```python
from build123d import *

# Parameters (mm, degrees)
BOSS_EXTRUDE1_DEPTH = 14
SKETCH2_R           = 2.75
CUT_EXTRUDE1_DEPTH  = 33.9


with BuildPart() as part:
    # Sketch1 → Boss-Extrude1 (new body)
    with BuildSketch(Plane.XY):
        with BuildLine():
            Line((-20.85, 6), (-20.85, 0))
            Line((-20.85, 0), (20.85, 0))
            Line((20.85, 0), (20.85, 6))
            Line((20.85, 6), (9, 6))
            Line((9, 6), (9, 32.9))
            Line((9, 32.9), (0.2, 32.9))
            Line((0.2, 32.9), (0.2, 24.445177921))
            ThreePointArc((0.2, 24.445177921), (3.004371815, 23.162909359), (4.15, 20.3))
            ThreePointArc((4.15, 20.3), (-2.862909359, 17.295628185), (-0.2, 24.445177921))
            Line((-0.2, 24.445177921), (-0.2, 32.9))
            Line((-0.2, 32.9), (-9, 32.9))
            Line((-9, 32.9), (-9, 6))
            Line((-9, 6), (-20.85, 6))
        make_face()
    extrude(amount=BOSS_EXTRUDE1_DEPTH)

    # Sketch2 → Cut-Extrude1 (cut, through all)
    with BuildSketch(Plane.XZ):
        with Locations((-15.85, 7)):
            Circle(SKETCH2_R)
        with Locations((15.85, 7)):
            Circle(SKETCH2_R)
    extrude(amount=-CUT_EXTRUDE1_DEPTH, mode=Mode.SUBTRACT)


solid = part.part
```
Read the model definition and answer for the solid it produces. Units are mm, in the model's axes. A direction names the side the tool comes from. Give positions to 0.01 mm unless a question says otherwise; leave off trailing zeros. Write each loop counter-clockwise with the first axis right and the second up, starting at its lowest first coordinate (ties: lowest second). Pieces come first, ordered by that corner, then holes. Notation, with made-up numbers: (32, -26) -> (90, -26) arc R18 ccw to (90, -9) -> close; hole circle Ø3 at (7, 0). An arc over 180 degrees is marked (long way). Answer in a Markdown table with one row per item.
1) A tool of negligible diameter and unlimited length cuts with its end or side. For faces 1 (the flat face through (0, 0, 7)), 2 (the flat face through (9, 19, 7)), 3 (the flat face through (-0.2, 29, 7)), 4 (the flat face through (-13.5, 6, 5.3)), from which of +Z, -Z, +X, -X, +Y, -Y can it reach the whole face along a straight path? Write none if from no direction.
Results list:
| item | result |
|---|---|
| face 1 | +Z, -Z, +X, -X, -Y |
| face 2 | +Z, -Z, +X, +Y |
| face 3 | +Z, -Z, +Y |
| face 4 | +Z, -Z, -X, +Y |
2) Each of these flat-tipped pins is pushed along its axis until it touches: pin 1 Ø4 at (y, z) = (28.5, 4) entering from -X; pin 2 Ø7 at (y, z) = (30, 7) entering from +X; pin 3 Ø3.5 at (x, z) = (-15.5, 9) entering from +Y. Where does it stop, or does it pass through?
Results list:
| item | result |
|---|---|
| pin 1 | x = -9 |
| pin 2 | x = 9 |
| pin 3 | y = 6 |
3) Section B-B on x = -15.85 is taken. Give the vertices of the cut face in (y, z).
Results list:
| item | result |
|---|---|
| outline | (0, 0) -> (6, 0) -> (6, 4.25) -> (0, 4.25) -> close; (0, 9.75) -> (6, 9.75) -> (6, 14) -> (0, 14) -> close |
4) Section C-C on z = 3 is taken. Give the vertices of the cut face in (x, y).
Results list:
| item | result |
|---|---|
| outline | (-20.85, 0) -> (20.85, 0) -> (20.85, 6) -> (9, 6) -> (9, 32.9) -> (0.2, 32.9) -> (0.2, 24.45) arc R4.15 cw (long way) to (-0.2, 24.45) -> (-0.2, 32.9) -> (-9, 32.9) -> (-9, 6) -> (-20.85, 6) -> close |
5) Straight lines are drawn through the part: line 1 (X direction, y = 25.5, z = 0.75); line 2 (Z direction, x = 15.85, y = 3.25); line 3 (Y direction, x = 0, z = 8.75). For each, find the intervals that lie inside material, in ascending order. Write a range as [from, to].
Results list:
| item | result |
|---|---|
| line 1 | [-9, -0.2], [0.2, 9] |
| line 2 | [0, 4.25], [9.75, 14] |
| line 3 | [0, 16.15] |
6) Section D-D on y = 13.5 is taken. Give the vertices of the cut face in (x, z).
Results list:
| item | result |
|---|---|
| outline | (-9, 0) -> (9, 0) -> (9, 14) -> (-9, 14) -> close |
7) Section A-A on y = 29.5 is taken. Give the vertices of the cut face in (x, z).
Results list:
| item | result |
|---|---|
| outline | (-9, 0) -> (-0.2, 0) -> (-0.2, 14) -> (-9, 14) -> close; (0.2, 0) -> (9, 0) -> (9, 14) -> (0.2, 14) -> close |
8) Determine the mould class of faces 5 (the flat face through (-5, 32.9, 7)), 6 (the flat face through (20.85, 3, 7)), 7 (the cylindrical face through (18.39, 2.96, 5.95)), 8 (the flat face through (-9, 20, 7)) for opening direction X: released by +X, released by -X, zero draft, split by the parting line, or undercut.
Results list:
| item | result |
|---|---|
| face 5 | zero draft |
| face 6 | released by +X |
| face 7 | undercut |
| face 8 | released by -X |
